Can you work these out from the model? Positions are in its coordinate system, mm. A direction names the side the tool comes from. Coordinates: 2 decimals unless noted, no trailing zeros. Loops run counter-clockwise (first coordinate to the right, second up) from the corner with the lowest first, then second, coordinate; pieces in that order, holes last. Notation, with made-up numbers: (39.25, -15.75) -> (85.25, -15.75) arc R24 cw to (85.25, 1.25) -> close; hole circle Ø10 at (-38, -11). An arc over 180 degrees is marked (long way). Use one line per item in the form item = value. Start each with the question number.
(1) Imagine slicing it at B-B (z = -0.25). List the corners of the cut face in (x, y) for me.
(2) On a 3-axis mill with a long thin cutter (end or side, diameter ignored), from which of +Z, -Z, +X, -X, +Y, -Y can I reach the whole of each face in a straight line? I mean faces 5 (the flat face through (-1, -25, 0)), 6 (the cylindrical face through (35, 0, 0)). Say none if no direction works.
(3) Imagine slicing it at A-A (x = -33). List the corners of the cut face in (y, z) for me.
(4) I need wall thicknesses on line 1 (Y direction, x = 18, z = -2.5); line 2 (X direction, y = -8.5, z = 2); line 3 (X direction, y = 8, z = 0.75). Which ranges of each line are inside material? Lowest first, please. Write a range as [from, to].
(5) Thinking about a two-plate mould opening in X: for faces 1 (the flat face through (-1, 11, -5)), 2 (the flat face through (50, 0, 0)), 3 (the flat face through (0, -10, 0)), 4 (the flat face through (0, 10, 0)), which applies, released by +X, released by -X, zero draft, split by the parting line, or undercut?
(6) Imagine slicing it at C-C (y = 0). List the corners of the cut face in (x, z) for me, plus the area to 3 significant figures.
```python
from build123d import *

# Parameters (mm, degrees)
SKETCH2_W       = 100
SKETCH2_H       = 50
BOX_DEPTH       = 5
HOLE_DEPTH      = 6
HOLE_DEPTH_BACK = 6


with BuildPart() as part:
    # Sketch2 → Box (new body, symmetric)
    with BuildSketch(Plane.XY):
        Rectangle(SKETCH2_W, SKETCH2_H)
    extrude(amount=BOX_DEPTH, both=True)

    # Sketch3 → Hole (cut, two sides)
    with BuildSketch(Plane.XY) as hole_sk:
        with BuildLine():
            Line((-25, 10), (25, 10))
            ThreePointArc((25, 10), (35, 0), (25, -10))
            Line((25, -10), (-25, -10))
            ThreePointArc((-25, -10), (-35, 0), (-25, 10))
        make_face()
    extrude(amount=HOLE_DEPTH, mode=Mode.SUBTRACT)
    extrude(hole_sk.sketch, amount=-HOLE_DEPTH_BACK, mode=Mode.SUBTRACT)


solid = part.part
```
Worked out:
q1.outline = (-50, -25) -> (50, -25) -> (50, 25) -> (-50, 25) -> close; hole (-25, -10) -> (25, -10) arc R10 ccw to (25, 10) -> (-25, 10) arc R10 ccw to start
q2.face_5 = +Z, -Z, +X, -X, -Y
q2.face_6 = +Z, -Z
q3.outline = (-25, -5) -> (-6, -5) -> (-6, 5) -> (-25, 5) -> close; (6, -5) -> (25, -5) -> (25, 5) -> (6, 5) -> close
q4.line_1 = [-25, -10], [10, 25]
q4.line_2 = [-50, -30.27], [30.27, 50]
q4.line_3 = [-50, -31], [31, 50]
q5.face_1 = zero draft
q5.face_2 = released by +X
q5.face_3 = undercut
q5.face_4 = undercut
q6.outline = (-50, -5) -> (-35, -5) -> (-35, 5) -> (-50, 5) -> close; (35, -5) -> (50, -5) -> (50, 5) -> (35, 5) -> close
q6.area = 300 mm2
